Answer from the drawing. Dimensions are ordinates in mm from the lowest x, y and z of the part. A direction names the side the tool comes from. Coordinates: 2 decimals unless noted, no trailing zeros. Order: outer loops, then holes, each group sorted by start corner. A loop starts at its lowest first (then second) coordinate and runs counter-clockwise, first axis right, second up.
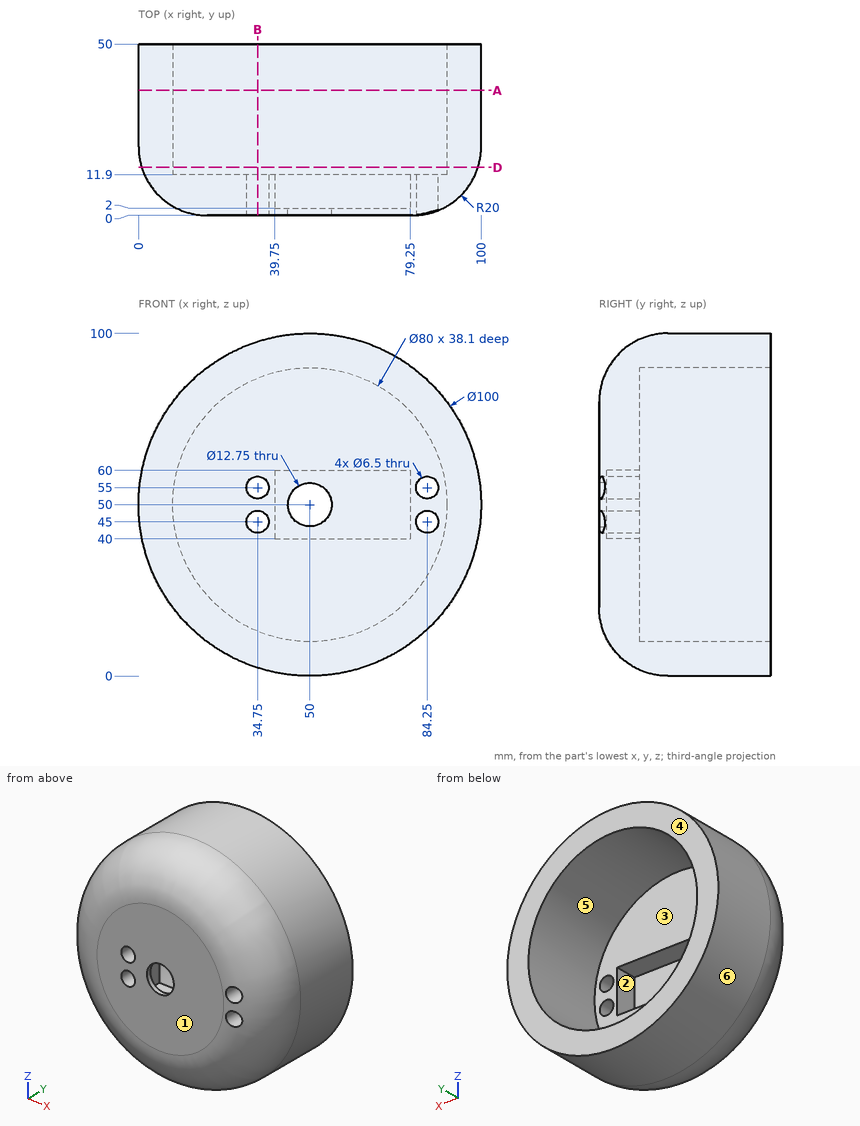
1. Flat-ended cylindrical pins translate along their axes: pin 1 (5 mm diameter, centred on x = 69.5, y = 9, fed in from +Z); pin 2 (5 mm diameter, centred on x = 55, y = 8, fed in from -Z); pin 3 (6 mm diameter, centred on y = 10, z = 45.5, fed in from +X); pin 4 (10.5 mm diameter, centred on x = 34.75, z = 55, fed in from -Y). Find the tip coordinate at first contact, or state that the pin passes through.
2. The part is cut by section B-B (x = 34.75). Count the separate pieces of the cut face and the enclosed holes in it, plus the area to 3 significant figures.
3. Consider probe 1 along Z at (x, y) = (84.25, 6); probe 2 along Z at (x, y) = (50, 25); probe 3 along Y at (x, z) = (31, 70.5). Determine where each line is inside the solid, lowest interval first.
4. The part is cut by section D-D (y = 14). Determine the outline of the cut face in (x, z).
5. The part is cut by section A-A (y = 36.5). Determine the outline of the cut face in (x, z).
6. The mould has two halves that part along Z. Classify the marked faces 3, 4, 5 and 6: released by +Z, released by -Z, zero draft, split by the parting line, or undercut.
7. For the marked faces 1 and 2, determine the directions among +Z, -Z, +X, -X, +Y, -Y from which every point of the face is accessible in a straight line to the end or side of a thin tool.
Worked out:
1. pin 1: stops at z = 94.35
1. pin 2: stops at z = 2.64
1. pin 3: stops at x = 98.56
1. pin 4: stops at y = 0
2. separate pieces: 3
2. enclosed holes: 0
2. area: 1,610 mm2
3. probe 1: z = 21.93 to 41.75, 48.25 to 51.75, 58.25 to 78.07
3. probe 2: z = 0 to 10, 90 to 100
3. probe 3: y = 0 to 11.9
4. outline: circle Ø98.16 at (50, 50); hole circle Ø80 at (50, 50)
5. outline: circle Ø100 at (50, 50); hole circle Ø80 at (50, 50)
6. face 3: undercut
6. face 4: zero draft
6. face 5: undercut
6. face 6: split by the parting line
7. face 1: +Z, -Z, +X, -X, -Y
7. face 2: +Y
